```python
from build123d import *

# Parameters (mm, degrees)
SKIZZE1_R                       = 40
AUFSATZ_LINEAR_AUSTRAGEN1_DEPTH = 4
SKIZZE2_W                       = 16
SKIZZE2_H                       = 45
AUFSATZ_LINEAR_AUSTRAGEN2_DEPTH = 17
SKIZZE3_W                       = 12
SKIZZE3_H                       = 22
AUFSATZ_LINEAR_AUSTRAGEN3_DEPTH = 27
SKIZZE4_R                       = 3.5
AUFSATZ_LINEAR_AUSTRAGEN4_DEPTH = 7


with BuildPart() as part:
    # Skizze1 → Aufsatz-Linear austragen1 (new body)
    with BuildSketch(Plane.XY):
        Circle(SKIZZE1_R)
    extrude(amount=AUFSATZ_LINEAR_AUSTRAGEN1_DEPTH)

    # Skizze2 → Aufsatz-Linear austragen2 (add)
    with BuildSketch(Plane.XY.offset(4)):
        with Locations((0, 5.5)):
            Rectangle(SKIZZE2_W, SKIZZE2_H)
    extrude(amount=AUFSATZ_LINEAR_AUSTRAGEN2_DEPTH)

    # Skizze3 → Aufsatz-Linear austragen3 (add)
    with BuildSketch(Plane.XY.offset(21)):
        with Locations((0, 5.5)):
            Rectangle(SKIZZE3_W, SKIZZE3_H)
    extrude(amount=AUFSATZ_LINEAR_AUSTRAGEN3_DEPTH)

    # Skizze4 → Aufsatz-Linear austragen4 (add)
    with BuildSketch(Plane.XY.offset(48)):
        Circle(SKIZZE4_R)
    extrude(amount=AUFSATZ_LINEAR_AUSTRAGEN4_DEPTH)


solid = part.part
```
Work out the finished part from the listing and answer in its coordinate system (mm). A direction names the side the tool comes from. Give positions to 0.01 mm unless a question says otherwise; leave off trailing zeros. Loops run counter-clockwise (first coordinate to the right, second up) from the corner with the lowest first, then second, coordinate; pieces in that order, holes last. Notation, with made-up numbers: (33, 34.5) -> (61, 34.5) arc R15 ccw to (61, 39.5) -> close; hole circle Ø11 at (28, -20.5). An arc over 180 degrees is marked (long way). Write item = value, one per line. Start each with the question number.
(1) Given pin 1 Ø1.5 at (x, z) = (-2.5, 7.5) entering from -Y; pin 2 Ø13 at (x, z) = (0, 13.5) entering from +Y; pin 3 Ø1 at (y, z) = (3.5, 10) entering from -X, each flat-ended and moving along its own axis, determine where each tip first touches the part or whether it passes through.
(2) Find the intervals of material crossed by probe 1 along Z at (x, y) = (-28, -3); probe 2 along X at (y, z) = (2.5, 13.5); probe 3 along Y at (x, z) = (5, 30), in increasing order. Write a range as from..to.
(3) Find section C-C on z = 6. Give the vertices of the cut face in (x, y), and give its area (3 significant figures).
(4) Find section B-B on y = 0. Give the vertices of the cut face in (x, z).
(5) Which of the six approach directions +Z, -Z, +X, -X, +Y, -Y give full straight-line access (tool end or side, diameter ignored) to faces 4 (the flat face through (8, 5, 12)), 5 (the flat face through (0, 16.5, 34)), 6 (the flat face through (-6, 5, 34))?
(6) The mould has two halves that part along Z. Classify faces 1 (the cylindrical face through (3.233, -1.341, 51.451)), 2 (the flat face through (-1, 1, 0)), 3 (the flat face through (0, 6, 48)): +Z half, -Z half, draft (parallel to the pull), parting line (faces both ways), or undercut.
(7) Find section A-A on x = 0. Give the vertices of the cut face in (y, z), and give its area (3 significant figures).
(8) Find section D-D on y = -14. Give the vertices of the cut face in (x, z), and give its area (3 significant figures).
From the geometry:
q1.pin_1 = -17
q1.pin_2 = 28
q1.pin_3 = -8
q2.probe_1 = 0..4
q2.probe_2 = -8..8
q2.probe_3 = -5.5..16.5
q3.outline = (-8, -17) -> (8, -17) -> (8, 28) -> (-8, 28) -> close
q3.area = 720 mm^2
q4.outline = (-40, 0) -> (40, 0) -> (40, 4) -> (8, 4) -> (8, 21) -> (6, 21) -> (6, 48) -> (3.5, 48) -> (3.5, 55) -> (-3.5, 55) -> (-3.5, 48) -> (-6, 48) -> (-6, 21) -> (-8, 21) -> (-8, 4) -> (-40, 4) -> close
q5.face_4 = +Z, +X, +Y, -Y
q5.face_5 = +Z, +X, -X, +Y
q5.face_6 = +Z, -X, +Y, -Y
q6.face_1 = draft
q6.face_2 = -Z half
q6.face_3 = +Z half
q7.outline = (-40, 0) -> (40, 0) -> (40, 4) -> (28, 4) -> (28, 21) -> (16.5, 21) -> (16.5, 48) -> (3.5, 48) -> (3.5, 55) -> (-3.5, 55) -> (-3.5, 48) -> (-5.5, 48) -> (-5.5, 21) -> (-17, 21) -> (-17, 4) -> (-40, 4) -> close
q7.area = 1,730 mm^2
q8.outline = (-37.47, 0) -> (37.47, 0) -> (37.47, 4) -> (8, 4) -> (8, 21) -> (-8, 21) -> (-8, 4) -> (-37.47, 4) -> close
q8.area = 572 mm^2
